Source: CAD feature listing. Evaluate the final solid. Frame: model axes, mm. Face numbers are marked on the shaded views. A direction names the side the tool comes from. Coordinates: 2 decimals unless noted, no trailing zeros. Loops run counter-clockwise (first coordinate to the right, second up) from the corner with the lowest first, then second, coordinate; pieces in that order, holes last.
Item 1: Pin query (flat end, axial travel): pin 1 Ø9.5 at (x, z) = (-11, -1.5) entering from -Y; pin 2 Ø7.5 at (x, z) = (31, -7.5) entering from +Y (3 decimals); pin 3 Ø1 at (y, z) = (8, 2) entering from +X (1 decimal); pin 4 Ø7 at (y, z) = (30, 7) entering from +X. Return the tip coordinate at first contact, or that it passes through.
Item 2: Line query: probe 1 along Z at (x, y) = (23, 11.5); probe 2 along Y at (x, z) = (33, -24) (3 decimals); probe 3 along X at (y, z) = (32.5, -0.5). Output: solid intervals per line, ascending.
Item 3: Section query C-C, the plane x = 9. Return the cut outline in (y, z) (3 decimals), then the cut area to 3 significant figures.
Item 4: Reachability of the marked faces 1, 2 and 3 from +Z, -Z, +X, -X, +Y, -Y: full face, straight path, thin tool, end or side. Return the list, or none.
Item 5: Section query A-A, the plane z = -6.35. Return the cut outline in (x, y) (3 decimals).
Item 6: Pull-direction query (X, two-part tool) for the marked faces 4, 5, 6 and 7; classes: +X half, -X half, draft (parallel to the pull), parting line (faces both ways), or undercut.
Item 7: Section query B-B, the plane y = 28. Return the cut outline in (x, z).
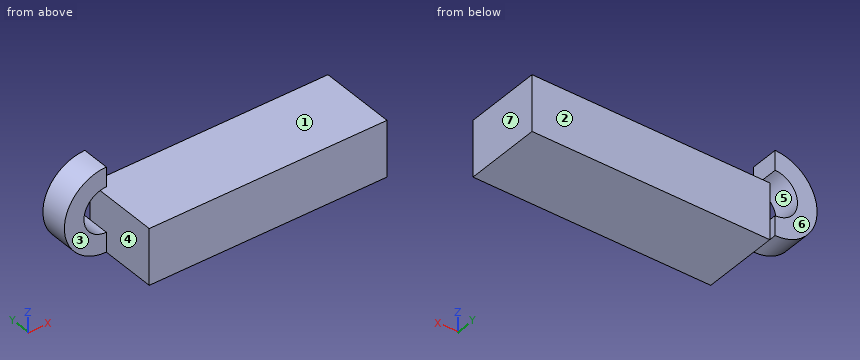
```python
from build123d import *

# Parameters (mm, degrees)
SKETCH1_W           = 107.95
SKETCH1_H           = 25.4
BOSS_EXTRUDE1_DEPTH = 34.925
BOSS_EXTRUDE2_DEPTH = 12.7


with BuildPart() as part:
    # Sketch1 → Boss-Extrude1 (new body)
    with BuildSketch(Plane(origin=(0, 0, 0), x_dir=(1, 0, 0), z_dir=(0, 1, 0))):
        with Locations((53.975, 12.7)):
            Rectangle(SKETCH1_W, SKETCH1_H)
    extrude(amount=BOSS_EXTRUDE1_DEPTH)

    # Sketch2 → Boss-Extrude2 (add)
    with BuildSketch(Plane(origin=(0, 25.4, 0), x_dir=(1, 0, 0), z_dir=(0, 1, 0))):
        with BuildLine():
            Line((0, 16.51), (0, 25.4))
            ThreePointArc((0, 25.4), (-19.05, 6.35), (0, -12.7))
            Line((0, -12.7), (0, -3.81))
            ThreePointArc((0, -3.81), (-10.16, 6.35), (0, 16.51))
        make_face()
    extrude(amount=BOSS_EXTRUDE2_DEPTH)


solid = part.part
```
Verdict:
1. pin 1: stops at y = 25.4
1. pin 2: stops at y = 34.925
1. pin 3: passes through
1. pin 4: stops at x = 0
2. probe 1: z = -25.4 to 0
2. probe 2: y = 0 to 34.925
2. probe 3: x = -18.13 to -8.31, 0 to 107.95
3. outline: (0, -25.4) - (34.925, -25.4) - (34.925, 0) - (0, 0) - close
3. area: 887 mm2
4. face 1: +Z, +X, +Y, -Y
4. face 2: +Z, -Z, +X, +Y
4. face 3: +Z, -Z, -X, -Y
5. outline: (-19.05, 25.4) - (-10.16, 25.4) - (-10.16, 38.1) - (-19.05, 38.1) - close; (0, 0) - (107.95, 0) - (107.95, 34.925) - (0, 34.925) - close
6. face 4: undercut
6. face 5: undercut
6. face 6: draft
6. face 7: +X half
7. outline: (0, -25.4) - (107.95, -25.4) - (107.95, 0) - (0, 0) - (0, -16.51) arc R10.16 cw to (0, 3.81) - (0, 12.7) arc R19.05 ccw to start
